```python
from build123d import *

# Parameters (mm, degrees)
BOSS_EXTRUDE1_DEPTH      = 1
BOSS_EXTRUDE1_DEPTH_BACK = 30
SKETCH1_R                = 400
SKETCH2_R                = 20
SKETCH2_W                = 40
SKETCH2_H                = 40
CUT_EXTRUDE1_DEPTH       = 10


with BuildPart() as part:
    # Sketch1 → Boss-Extrude1 (new, two sides: drawn at the far end of the back side and taken through both)
    with BuildSketch(Plane(origin=(0, 0, 0), x_dir=(1, 0, 0), z_dir=(0, 1, 0)).offset(-BOSS_EXTRUDE1_DEPTH_BACK)):
        with Locations(Location((0, 0, 0), (0, 0, 270))):
            Circle(SKETCH1_R)
    extrude(amount=BOSS_EXTRUDE1_DEPTH + BOSS_EXTRUDE1_DEPTH_BACK)

    # Sketch2 → Cut-Extrude1 (cut)
    with BuildSketch(Plane(origin=(0, 1, 0), x_dir=(1, 0, 0), z_dir=(0, 1, 0))):
        with Locations(Location((-360, 0, 0), (0, 0, 270))):
            Circle(SKETCH2_R)
        with Locations(Location((360, 0, 0), (0, 0, 270))):
            Circle(SKETCH2_R)
        with Locations((0, 360)):
            Rectangle(SKETCH2_W, SKETCH2_H)
    extrude(amount=-CUT_EXTRUDE1_DEPTH, mode=Mode.SUBTRACT)


solid = part.part
```
Design review of the part built by this model. Coordinates are the model's own, in mm. A direction names the side the tool comes from. Coordinates: 2 decimals unless noted, no trailing zeros. Order: outer loops, then holes, each group sorted by start corner. A loop starts at its lowest first (then second) coordinate and runs counter-clockwise, first axis right, second up.
1) Wall thickness on line 1 along X through (y, z) = (-6.5, 0); line 2 along X through (y, z) = (-1, -8); line 3 along Z through (x, y) = (326, -7): over which ranges is each line inside the solid? List them lowest first.
2) Take a section at D-D, the plane x = -360. Give the boundary of the cut face in (y, z).
3) Take a section at C-C, the plane y = -16. Give the boundary of the cut face in (x, z), and give its area (3 significant figures).
4) Clearance check with flat-ended pins moving along their axes: pin 1 (12 mm diameter, centred on x = 360.5, z = 0, fed in from +Y); pin 2 (5 mm diameter, centred on y = -9, z = -32, fed in from +X); pin 3 (1.5 mm diameter, centred on x = 171, y = -17, fed in from -Z). State where each tip first meets the part, or that it passes through.
5) For faces 5 (the flat face through (6, 1, -6)), 6 (the flat face through (-360, -9, 0)), list the 3-axis set-ups (+Z, -Z, +X, -X, +Y, -Y) from which the entire face can be reached by the end or side of a thin tool; tool diameter is ignored.
6) Take a section at B-B, the plane z = 0. Give the boundary of the cut face in (x, y), and give its area (3 significant figures).
7) Mouldability with a two-part tool opening along Z and no side actions: class faces 1 (the cylindrical face through (-379.524, -3.93, -4.336)), 2 (the cylindrical face through (120.15, -14.72, 381.53)), 3 (the flat face through (0, -9, -360)), 4 (the flat face through (6, -30, -6)) as +Z half, -Z half, draft (parallel to the pull), parting line (faces both ways), or undercut.
8) Take a section at A-A, the plane x = 0. Give the boundary of the cut face in (y, z), and give its area (3 significant figures).
Returned:
1. line 1: x = -400 to -380, -340 to 340, 380 to 400
1. line 2: x = -399.92 to -378.33, -341.67 to 341.67, 378.33 to 399.92
1. line 3: z = -231.78 to 231.78
2. outline: (-30, -174.36) - (1, -174.36) - (1, -20) - (-9, -20) - (-9, 20) - (1, 20) - (1, 174.36) - (-30, 174.36) - close
3. outline: circle Ø800 at (0, 0)
3. area: 503,000 mm2
4. pin 1: stops at y = -9
4. pin 2: stops at x = 398.91
4. pin 3: stops at z = -361.96
5. face 5: +Z, -Z, +X, -X, +Y
5. face 6: +Y
6. outline: (-400, -30) - (400, -30) - (400, 1) - (380, 1) - (380, -9) - (340, -9) - (340, 1) - (-340, 1) - (-340, -9) - (-380, -9) - (-380, 1) - (-400, 1) - close
6. area: 24,000 mm2
7. face 1: undercut
7. face 2: parting line
7. face 3: undercut
7. face 4: draft
8. outline: (-30, -400) - (1, -400) - (1, -380) - (-9, -380) - (-9, -340) - (1, -340) - (1, 400) - (-30, 400) - close
8. area: 24,400 mm2
